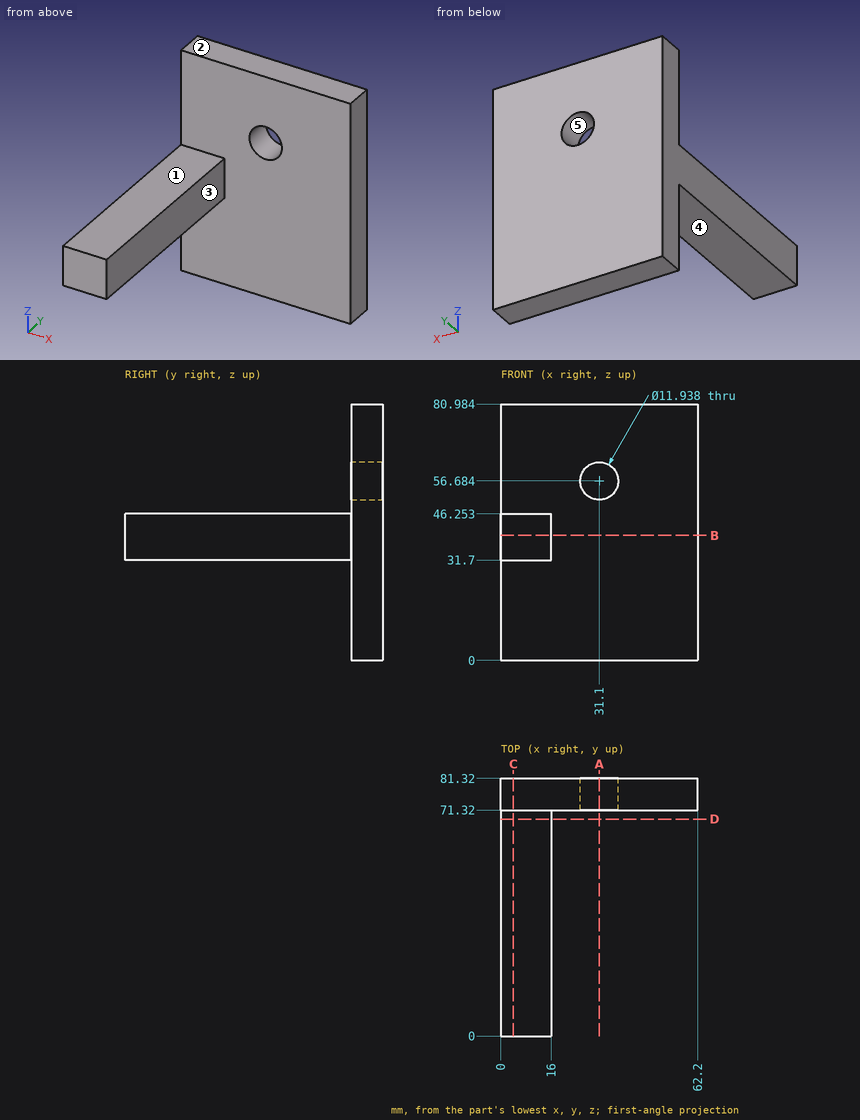
Can you work these out from the drawing? Everything is in mm from the part's minimum corner. A direction names the side the tool comes from. Give positions to 0.01 mm unless a question says otherwise; leave off trailing zeros. Loops run counter-clockwise (first coordinate to the right, second up) from the corner with the lowest first, then second, coordinate; pieces in that order, holes last. Notation, with made-up numbers: M 58.5,2.25 L 104.5,2.25 A12 ccw 104.5,8.25 Z; hole C -36,-31.5 d2. An arc over 180 degrees is marked long. Use CSV: the item, a comma, the result in double quotes. Start each with the question number.
1. On a 3-axis mill with a long thin cutter (end or side, diameter ignored), from which of +Z, -Z, +X, -X, +Y, -Y can I reach the whole of each face in a straight line? I mean the marked faces 1 and 2. Say none if no direction works.
2. Imagine slicing it at C-C, the plane x = 4. Write out the boundary of the cut face in (y, z), plus the area to 3 significant figures.
3. Imagine slicing it at A-A, the plane x = 31.1. Write out the boundary of the cut face in (y, z) (1 decimal).
4. Imagine slicing it at B-B, the plane z = 39.5. Write out the boundary of the cut face in (x, y).
5. If we mould it in two halves opening along X, with no side actions, what happens to the marked faces 3, 4 and 5? For each: released by +X, released by -X, zero draft, split by the parting line, or undercut.
6. If I drill on L1, parallel to Z at x = 31, y = 78; L2, parallel to Y at x = 34, z = 32.5; L3, parallel to Z at x = 14, y = 53, over which ranges is the centre line in solid material (lowest first)?
7. Imagine slicing it at D-D, the plane y = 68.5. Write out the boundary of the cut face in (x, z).
8. For P1, Ø11.5, axis at y = 38.5, z = 36, coming from the +X side; P2, Ø18.5, axis at x = 40, z = 51.5, coming from the -Y side; P3, Ø15.5, axis at x = 31.1, z = 56.68, coming from the +Y side; P4, Ø13, axis at x = 7, y = 48.5, coming from the -Z side, each with a flat end and sliding along its axis, tell me the tip position at first contact or that it passes through.
Response values:
1,face 1,"+Z, +X, -X, -Y"
1,face 2,"+Z, +X, -X, +Y, -Y"
2,outline,"M 0,31.7 L 71.32,31.7 L 71.32,0 L 81.32,0 L 81.32,80.98 L 71.32,80.98 L 71.32,46.25 L 0,46.25 Z"
2,area,"1,850 mm^2"
3,outline,"M 71.3,0 L 81.3,0 L 81.3,50.7 L 71.3,50.7 Z; M 71.3,62.7 L 81.3,62.7 L 81.3,81 L 71.3,81 Z"
4,outline,"M 0,0 L 16,0 L 16,71.32 L 62.2,71.32 L 62.2,81.32 L 0,81.32 Z"
5,face 3,"released by +X"
5,face 4,"zero draft"
5,face 5,"undercut"
6,L1,"0 to 50.72, 62.65 to 80.98"
6,L2,"71.32 to 81.32"
6,L3,"31.7 to 46.25"
7,outline,"M 0,31.7 L 16,31.7 L 16,46.25 L 0,46.25 Z"
8,P1,"x = 16"
8,P2,"y = 71.32"
8,P3,"y = 81.32"
8,P4,"z = 31.7"
